The model under review builds one solid part; all positions refer to its coordinate system, in mm. Give positions to 0.01 mm unless a question says otherwise; leave off trailing zeros. Write each loop counter-clockwise with the first axis right and the second up, starting at its lowest first coordinate (ties: lowest second). Pieces come first, ordered by that corner, then holes.
Autodesk Inventor part; units mm, degrees
ref_plane "YZ Plane" through (0, 0, 0) normal (1, 0, 0) x (0, 1, 0)
ref_plane "XZ Plane" through (0, 0, 0) normal (0, 1, 0) x (-1, 0, 0)
ref_plane "XY Plane" through (0, 0, 0) normal (0, 0, 1) x (1, 0, 0)
sketch "Sketch1" plane through (0, 0, 0) normal (0, 0, 1) x (1, 0, 0)
  line L0 (18.2242, 0) -> (206.7758, 0)
  line L1 (-6.65, 150) -> (231.65, 150)
  line L2 (-6.65, 150) -> (-0.8071, 18.2063)
  line L3 (225.8071, 18.2063) -> (231.65, 150)
  arc A0 (-0.8071, 18.2063) -> (18.2242, 0) centre (18.2242, 19.05) ccw
  arc A1 (206.7758, 0) -> (225.8071, 18.2063) centre (206.7758, 19.05) ccw
  circle A2 centre (112.5, 41.275) radius 22.225
  point P0 (0, 0)
  point P1 (225, 0)
  point P2 (112.5, 0)
  point P3 (112.5, 150)
  dimension "d0" = 225
  dimension "d1" = 150
  dimension "d2" = 238.3
  dimension "d4" = 19.05
  dimension "d11" = 0
  dimension "d12" = 44.45
  dimension "d13" = 41.275
extrude "Extrusion1" add sketch "Sketch1" along normal blind 25.4
sketch "Sketch2" plane through (0, 0, 25.4) normal (0, 0, 1) x (1, 0, 0)
  line L0 (243.0343, 163.5066) -> (27.3006, 163.5066)
  line L1 (27.3006, 163.5066) -> (27.3006, 18.9917)
  line L2 (27.3006, 18.9917) -> (243.0343, 18.9917)
  line L3 (243.0343, 18.9917) -> (243.0343, 163.5066)
  line L4 (27.1522, 18.9917) -> (243.0343, 18.9917)
  line L5 (243.0343, 18.9917) -> (243.0343, -17.0628)
  line L6 (243.0343, -17.0628) -> (27.1522, -17.0628)
  line L7 (27.1522, -17.0628) -> (27.1522, 18.9917)
  point P0 (0, 0)
extrude "Test" [suppressed]
properties part number "Divider_3DPrint"
1) Insertion check: pin 1 (6 mm diameter, centred on x = 54.5, z = 10, fed in from -Y); pin 2 (8 mm diameter, centred on y = 74.5, z = 20.5, fed in from -X). Each pin has a flat end and moves straight along its axis. Give the tip position at first contact, or say it passes through.
2) The part is to be moulded in two halves that separate along X. For faces 1 (the flat face through (111, 0, 13)), 2 (the cylindrical face through (5.203, 5.145, 12.522)), 3 (the cylindrical face through (133.03, 49.79, 12.52)), say which applies: +X half, -X half, draft (parallel to the pull), parting line (faces both ways), or undercut.
3) Consider section C-C, the plane z = 10.25. Give the boundary of the cut face in (x, y) (3 decimals).
4) Consider section A-A, the plane x = 112.5. Give the boundary of the cut face in (y, z), then the cut area to 3 significant figures.
5) To check wall thickness, follow probe 1 along Y at (x, z) = (112.5, 14.25); probe 2 along X at (y, z) = (42, 2.5); probe 3 along Y at (x, z) = (125.5, 18). State the ranges of each line that lie inside material, in increasing order.
6) Consider section B-B, the plane y = 60.5. Give the boundary of the cut face in (x, z).
7) Consider section D-D, the plane y = 98. Give the boundary of the cut face in (x, z), then the cut area to 3 significant figures.
Answer block:
1. pin 1: stops at y = 0
1. pin 2: stops at x = -3.48
2. face 1: draft
2. face 2: -X half
2. face 3: undercut
3. outline: (-6.65, 150) - (-0.807, 18.206) arc R19.05 ccw to (18.224, 0) - (206.776, 0) arc R19.05 ccw to (225.807, 18.206) - (231.65, 150) - close; hole circle Ø44.45 at (112.5, 41.275)
4. outline: (0, 0) - (19.05, 0) - (19.05, 25.4) - (0, 25.4) - close; (63.5, 0) - (150, 0) - (150, 25.4) - (63.5, 25.4) - close
4. area: 2,680 mm2
5. probe 1: y = 0 to 19.05, 63.5 to 150
5. probe 2: x = -1.86 to 90.29, 134.71 to 226.86
5. probe 3: y = 0 to 23.25, 59.3 to 150
6. outline: (-2.68, 0) - (101.35, 0) - (101.35, 25.4) - (-2.68, 25.4) - close; (123.65, 0) - (227.68, 0) - (227.68, 25.4) - (123.65, 25.4) - close
7. outline: (-4.34, 0) - (229.34, 0) - (229.34, 25.4) - (-4.34, 25.4) - close
7. area: 5,940 mm2
